For this review, use the dimensioned drawing (mm, ordinates from the lowest corner) and the shaded views. A direction names the side the tool comes from. Give positions to 0.01 mm unless a question says otherwise; leave off trailing zeros. Loops run counter-clockwise (first coordinate to the right, second up) from the corner with the lowest first, then second, coordinate; pieces in that order, holes last. Notation, with made-up numbers: M -29,56.25 L 20,56.25 A30 ccw 20,81.25 Z; hole C -1.5,-28.75 d8. An arc over 180 degrees is marked long. Use CSV: the item, a comma, the result in double quotes. Start each with the question number.
1. Insertion check: P1, Ø17, axis at x = 122.5, y = 23.5, coming from the -Z side; P2, Ø3, axis at x = 31, y = 222, coming from the -Z side; P3, Ø6, axis at y = 65, z = 465.5, coming from the +X side; P4, Ø8, axis at y = 101, z = 90.5, coming from the -X side. Each pin has a flat end and moves straight along its axis. Give the tip position at first contact, or say it passes through.
2. Take a section at A-A, the plane x = 91. Write out the cut boundary in (y, z).
3. Take a section at B-B, the plane y = 31. Write out the cut boundary in (x, z).
4. To check wall thickness, follow line 1 (Y direction, x = 64.5, z = 451.5); line 2 (X direction, y = 166, z = 185); line 3 (Y direction, x = 55.5, z = 370). State the ranges of each line that lie inside material, in increasing order. Write a range as [from, to].
5. Tool access review of the marked faces 1, 2 and 3: name each direction out of +Z, -Z, +X, -X, +Y, -Y from which nothing blocks a thin tool from reaching the whole face with its end or side.
6. Take a section at C-C, the plane z = 125. Write out the cut boundary in (x, y).
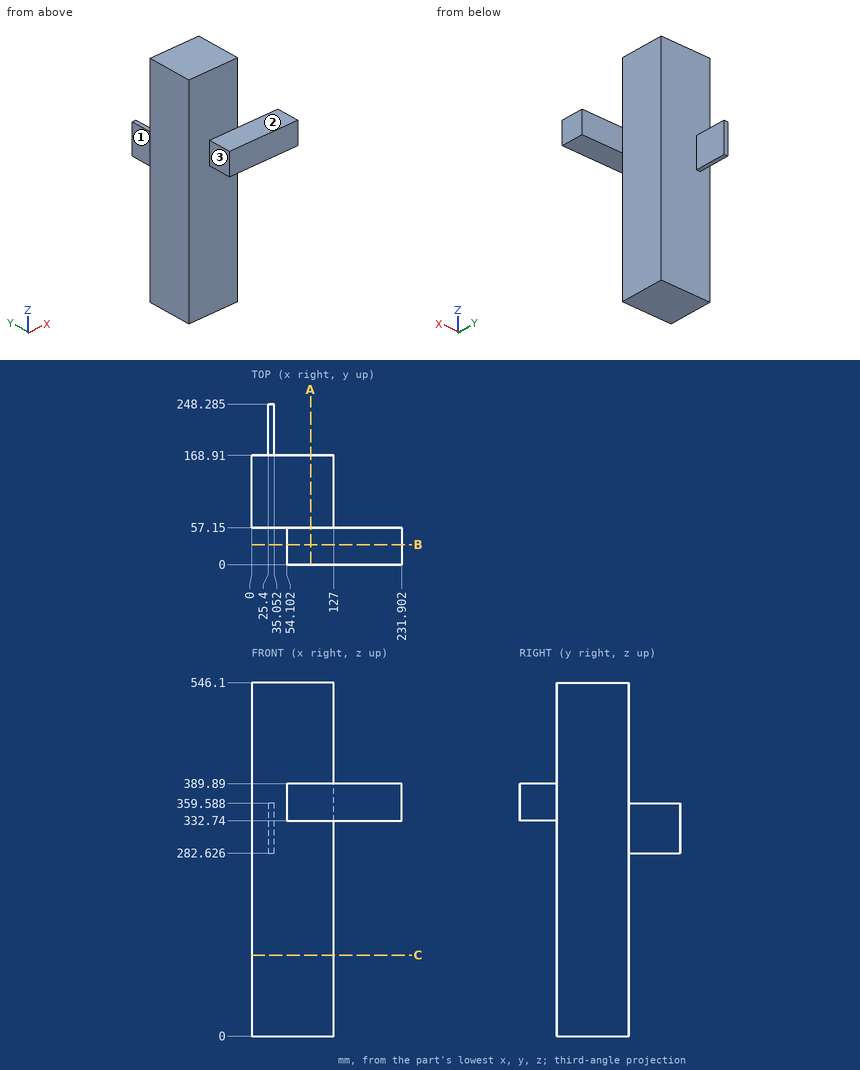
Result set:
1,P1,"z = 332.74"
1,P2,"z = 282.63"
1,P3,"x = 127"
1,P4,"x = 0"
2,outline,"M 0,332.74 L 57.15,332.74 L 57.15,0 L 168.91,0 L 168.91,546.1 L 57.15,546.1 L 57.15,389.89 L 0,389.89 Z"
3,outline,"M 54.1,332.74 L 231.9,332.74 L 231.9,389.89 L 54.1,389.89 Z"
4,line 1,"[57.15, 168.91]"
4,line 2,"[0, 127]"
4,line 3,"[0, 168.91]"
5,face 1,"+Z, -Z, -X, +Y"
5,face 2,"+Z, +X, -X, -Y"
5,face 3,"+Z, -Z, -X, -Y"
6,outline,"M 0,57.15 L 127,57.15 L 127,168.91 L 0,168.91 Z"
